Geometry: final body of the model. Coordinates: model frame, mm. A direction names the side the tool comes from. Round coordinates to 2 decimals unless told otherwise and drop trailing zeros. Answer in a Markdown table with one row per item.
```python
from build123d import *

# Parameters (mm, degrees)
SKETCH1_R           = 0.35
BOSS_EXTRUDE1_DEPTH = 0.4


with BuildPart() as part:
    # Sketch1 → Boss-Extrude1 (new body)
    with BuildSketch(Plane.XY):
        with BuildLine():
            Line((1.717219809, 2.640768094), (2.689842019, 3.094309279))
            Line((2.689842019, 3.094309279), (2.507060643, 3.38396102))
            Line((2.507060643, 3.38396102), (2.4713431, 3.33575047))
            ThreePointArc((2.4713431, 3.33575047), (2.524919075, 3.194040009), (2.418160882, 3.086546159))
            ThreePointArc((2.418160882, 3.086546159), (1.538245687, 2.989134777), (0.657689973, 3.080575255))
            ThreePointArc((0.657689973, 3.080575255), (0.576375294, 3.096819581), (0.494661207, 3.110917918))
            Line((0.494661207, 3.110917918), (1.198723989, 3.920849499))
            Line((1.198723989, 3.920849499), (0.913932917, 4.111115649))
            Line((0.913932917, 4.111115649), (0.900912315, 4.052545486))
            ThreePointArc((0.900912315, 4.052545486), (1.007495241, 3.94487785), (0.953688466, 3.803254863))
            ThreePointArc((0.953688466, 3.803254863), (0.189466715, 3.356371385), (-0.65215315, 3.081752143))
            ThreePointArc((-0.65215315, 3.081752143), (-0.733044969, 3.063518414), (-0.813428812, 3.043161771))
            Line((-0.813428812, 3.043161771), (-0.499664308, 4.069439222))
            Line((-0.499664308, 4.069439222), (-0.837222113, 4.127421033))
            Line((-0.837222113, 4.127421033), (-0.825294394, 4.068618571))
            ThreePointArc((-0.825294394, 4.068618571), (-0.684133674, 4.013610473), (-0.675685349, 3.862346249))
            ThreePointArc((-0.675685349, 3.862346249), (-1.192072773, 3.143260888), (-1.84923307, 2.550066088))
            ThreePointArc((-1.84923307, 2.550066088), (-1.915715097, 2.500507082), (-1.9808696, 2.449215309))
            Line((-1.9808696, 2.449215309), (-2.111656107, 3.514385933))
            Line((-2.111656107, 3.514385933), (-2.443613834, 3.430057825))
            Line((-2.443613834, 3.430057825), (-2.408800204, 3.381190544))
            ThreePointArc((-2.408800204, 3.381190544), (-2.25746966, 3.388353383), (-2.18822703, 3.253602881))
            ThreePointArc((-2.18822703, 3.253602881), (-2.367492049, 2.386652029), (-2.726563791, 1.577450441))
            ThreePointArc((-2.726563791, 1.577450441), (-2.767140682, 1.505135359), (-2.805800038, 1.431777269))
            Line((-2.805800038, 1.431777269), (-3.358523382, 2.351663389))
            Line((-3.358523382, 2.351663389), (-3.627482524, 2.139606457))
            Line((-3.627482524, 2.139606457), (-3.575802576, 2.109123954))
            ThreePointArc((-3.575802576, 2.109123954), (-3.440468635, 2.17721921), (-3.322404377, 2.082282016))
            ThreePointArc((-3.322404377, 2.082282016), (-3.133550441, 1.217369352), (-3.132446863, 0.332079281))
            ThreePointArc((-3.132446863, 0.332079281), (-3.140102504, 0.249512058), (-3.14558216, 0.166771932))
            Line((-3.14558216, 0.166771932), (-4.024671452, 0.782316881))
            Line((-4.024671452, 0.782316881), (-4.18412653, 0.479197696))
            Line((-4.18412653, 0.479197696), (-4.124516198, 0.472370671))
            ThreePointArc((-4.124516198, 0.472370671), (-4.028579326, 0.589624057), (-3.882107824, 0.550915675))
            ThreePointArc((-3.882107824, 0.550915675), (-3.357789496, -0.162407546), (-2.996701415, -0.970711403))
            ThreePointArc((-2.996701415, -0.970711403), (-2.970112076, -1.049254144), (-2.941464549, -1.127069787))
            Line((-2.941464549, -1.127069787), (-3.994917266, -0.922299323))
            Line((-3.994917266, -0.922299323), (-4.017297048, -1.264068701))
            Line((-4.017297048, -1.264068701), (-3.960063499, -1.246059791))
            ThreePointArc((-3.960063499, -1.246059791), (-3.920112054, -1.099922453), (-3.770559561, -1.075708992))
            ThreePointArc((-3.770559561, -1.075708992), (-3.001436241, -1.514102704), (-2.342799068, -2.105657267))
            ThreePointArc((-2.342799068, -2.105657267), (-2.286562287, -2.166594772), (-2.228740996, -2.226030901))
            Line((-2.228740996, -2.226030901), (-3.274405591, -2.467441595))
            Line((-3.274405591, -2.467441595), (-3.15584041, -2.788766135))
            Line((-3.15584041, -2.788766135), (-3.110879844, -2.749035196))
            ThreePointArc((-3.110879844, -2.749035196), (-3.133821794, -2.599282378), (-3.007047295, -2.516333802))
            ThreePointArc((-3.007047295, -2.516333802), (-2.126107394, -2.603995748), (-1.283805479, -2.87651586))
            ThreePointArc((-1.283805479, -2.87651586), (-1.207645106, -2.909311482), (-1.130647877, -2.940091049))
            Line((-1.130647877, -2.940091049), (-1.987719443, -3.585940799))
            Line((-1.987719443, -3.585940799), (-1.748710296, -3.83126057))
            Line((-1.748710296, -3.83126057), (-1.723796804, -3.776677441))
            ThreePointArc((-1.723796804, -3.776677441), (-1.805665276, -3.649202766), (-1.723589234, -3.521861637))
            ThreePointArc((-1.723589234, -3.521861637), (-0.883155263, -3.243634272), (-0.002830259, -3.149998729))
            ThreePointArc((-0.002830259, -3.149998729), (0.080084884, -3.148981805), (0.162944532, -3.145782745))
            Line((0.162944532, -3.145782745), (-0.357338545, -4.084398262))
            Line((-0.357338545, -4.084398262), (-0.039212284, -4.211295246))
            Line((-0.039212284, -4.211295246), (-0.038653636, -4.151297847))
            ThreePointArc((-0.038653636, -4.151297847), (-0.165292828, -4.068142844), (-0.142106936, -3.9184276))
            ThreePointArc((-0.142106936, -3.9184276), (0.512502436, -3.322418962), (1.278634338, -2.8788182))
            ThreePointArc((1.278634338, -2.8788182), (1.353967471, -2.844164568), (1.42836235, -2.807540026))
            Line((1.42836235, -2.807540026), (1.334829433, -3.87662616))
            Line((1.334829433, -3.87662616), (1.677065887, -3.863158716))
            Line((1.677065887, -3.863158716), (1.653173097, -3.808121141))
            ThreePointArc((1.653173097, -3.808121141), (1.503660251, -3.783664066), (1.463946943, -3.637461833))
            ThreePointArc((1.463946943, -3.637461833), (1.819543808, -2.826727231), (2.339011442, -2.109863852))
            ThreePointArc((2.339011442, -2.109863852), (2.393736781, -2.047565438), (2.446803342, -1.98384813))
            Line((2.446803342, -1.98384813), (2.796193276, -2.998550177))
            Line((2.796193276, -2.998550177), (3.103364131, -2.847046948))
            Line((3.103364131, -2.847046948), (3.059151183, -2.806485695))
            ThreePointArc((3.059151183, -2.806485695), (2.912616813, -2.844955398), (2.816871095, -2.72754587))
            ThreePointArc((2.816871095, -2.72754587), (2.811969526, -1.842268681), (2.994952219, -0.976094876))
            ThreePointArc((2.994952219, -0.976094876), (3.019607256, -0.896923642), (3.042169808, -0.81713087))
            Line((3.042169808, -0.81713087), (3.774069899, -1.601997627))
            Line((3.774069899, -1.601997627), (3.993062523, -1.338654898))
            Line((3.993062523, -1.338654898), (3.936174238, -1.319583375))
            ThreePointArc((3.936174238, -1.319583375), (3.817955468, -1.414328096), (3.682732645, -1.346012447))
            ThreePointArc((3.682732645, -1.346012447), (3.318180166, -0.53926514), (3.133038549, 0.326449772))
            ThreePointArc((3.133038549, 0.326449772), (3.123360204, 0.4088044), (3.111517477, 0.490875741))
            Line((3.111517477, 0.490875741), (4.09937555, 0.071554866))
            Line((4.09937555, 0.071554866), (4.19232413, 0.401202745))
            Line((4.19232413, 0.401202745), (4.132597008, 0.395486898))
            ThreePointArc((4.132597008, 0.395486898), (4.063134937, 0.260849383), (3.911816263, 0.268258756))
            ThreePointArc((3.911816263, 0.268258756), (3.250647311, 0.856982243), (2.72939405, 1.572548288))
            ThreePointArc((2.72939405, 1.572548288), (2.687055797, 1.643846447), (2.642855506, 1.714005476))
            Line((2.642855506, 1.714005476), (3.715861927, 1.732734873))
            Line((3.715861927, 1.732734873), (3.666694808, 2.071688789))
            Line((3.666694808, 2.071688789), (3.614456212, 2.042173893))
            ThreePointArc((3.614456212, 2.042173893), (3.605761463, 1.890923633), (3.464511313, 1.836145584))
            ThreePointArc((3.464511313, 1.836145584), (2.621048005, 2.105049611), (1.853812525, 2.546738919))
            ThreePointArc((1.853812525, 2.546738919), (1.786135033, 2.59465251), (1.717219809, 2.640768094))
        make_face()
        with BuildLine():
            ThreePointArc((-0.831790238, -0.175), (-0.601040764, -0.601040764), (-0.175, -0.831790238))
            Line((-0.175, -0.831790238), (-0.175, -2.794525899))
            ThreePointArc((-0.175, -2.794525899), (-1.979898987, -1.979898987), (-2.794525899, -0.175))
            Line((-2.794525899, -0.175), (-0.831790238, -0.175))
        make_face(mode=Mode.SUBTRACT)
        with BuildLine():
            ThreePointArc((0.175, -0.831790238), (0.601040764, -0.601040764), (0.831790238, -0.175))
            Line((0.831790238, -0.175), (2.794525899, -0.175))
            ThreePointArc((2.794525899, -0.175), (1.979898987, -1.979898987), (0.175, -2.794525899))
            Line((0.175, -2.794525899), (0.175, -0.831790238))
        make_face(mode=Mode.SUBTRACT)
        with BuildLine():
            Line((-0.175, 2.794525899), (-0.175, 0.831790238))
            ThreePointArc((-0.175, 0.831790238), (-0.601040764, 0.601040764), (-0.831790238, 0.175))
            Line((-0.831790238, 0.175), (-2.794525899, 0.175))
            ThreePointArc((-2.794525899, 0.175), (-1.979898987, 1.979898987), (-0.175, 2.794525899))
        make_face(mode=Mode.SUBTRACT)
        Circle(SKETCH1_R, mode=Mode.SUBTRACT)
        with BuildLine():
            Line((2.794525899, 0.175), (0.831790238, 0.175))
            ThreePointArc((0.831790238, 0.175), (0.601040764, 0.601040764), (0.175, 0.831790238))
            Line((0.175, 0.831790238), (0.175, 2.794525899))
            ThreePointArc((0.175, 2.794525899), (1.979898987, 1.979898987), (2.794525899, 0.175))
        make_face(mode=Mode.SUBTRACT)
    extrude(amount=BOSS_EXTRUDE1_DEPTH)


solid = part.part
```
Item 1: Draft query along Y for faces 1 (the face through (-1.184, 3.153, 0.197)), 2 (the face through (0, 1, 0.4)). Return one class per face: pulls with the +Y half, pulls with the -Y half, needs draft (parallel to the pull), parting line crosses it, or undercut.
Answer:
| item | result |
|---|---|
| face 1 | undercut |
| face 2 | needs draft |
Item 2: Reachability of faces 3 (the face through (0, 1, 0)), 4 (the face through (-3.01, -1.51, 0.2)) from +Z, -Z, +X, -X, +Y, -Y: full face, straight path, thin tool, end or side. Return the list, or none.
Answer:
| item | result |
|---|---|
| face 3 | -Z, +X, -X, +Y, -Y |
| face 4 | +Z, -Z |
Item 3: Line query: probe 1 along Y at (x, z) = (0, 0.35); probe 2 along Y at (x, z) = (1.25, 0.05) (1 decimal); probe 3 along Y at (x, z) = (0.75, 0.1). Output: solid intervals per line, ascending. Write a range as [from, to].
Answer:
| item | result |
|---|---|
| probe 1 | y = [-3.77, -3.44], [-3.15, -0.35], [0.35, 3.28] |
| probe 2 | y = [-2.9, -2.5], [-0.2, 0.2], [2.5, 3] |
| probe 3 | y = [-3.16, -2.7], [-0.4, 0.4], [2.7, 3.06], [3.4, 3.66] |
Item 4: Pin query (flat end, axial travel): pin 1 Ø2 at (x, y) = (2, -1) entering from -Z. Return the tip coordinate at first contact, or that it passes through.
Answer:
| item | result |
|---|---|
| pin 1 | stops at z = 0 |
Item 5: Cut plane A-A (z = 0.1). Count the separate pieces of the cut face and the enclosed holes in it, then the cut area to 3 significant figures.
Answer:
| item | result |
|---|---|
| separate pieces | 1 |
| enclosed holes | 5 |
| area | 16.0 mm² |
